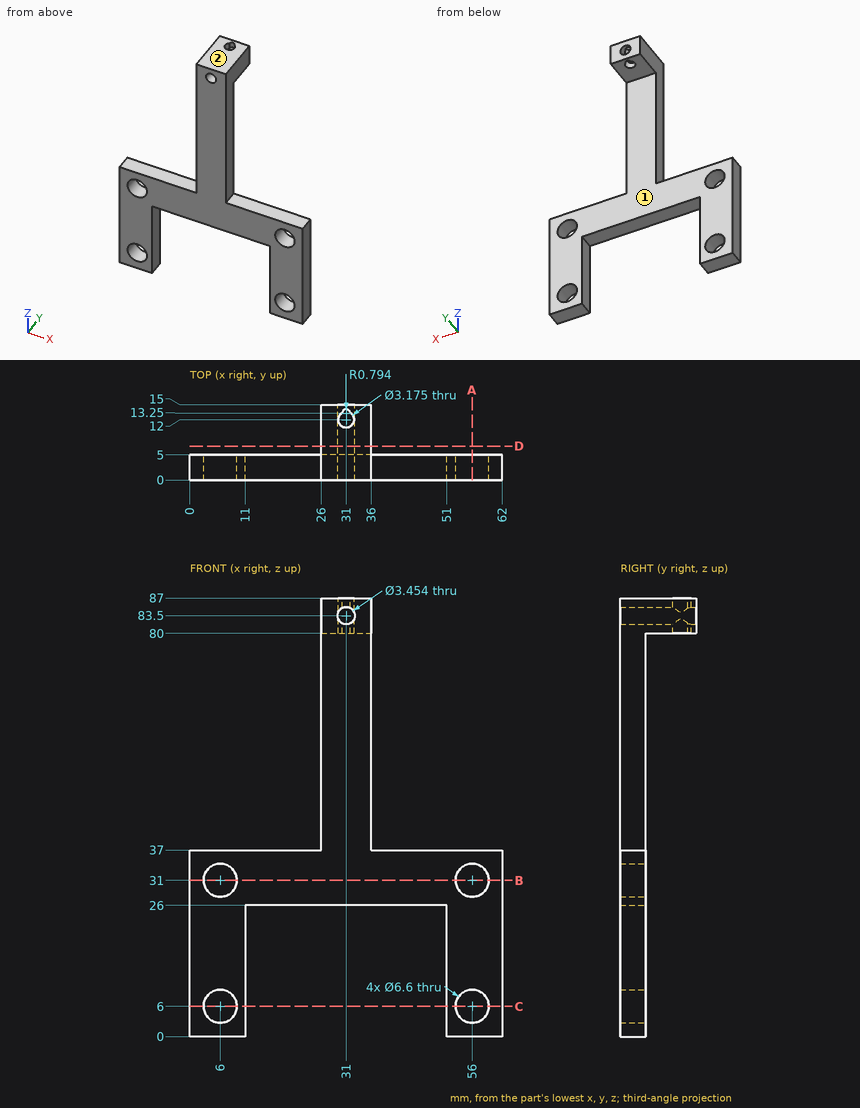
Design review of the part shown in the three views and the two pictorial views. Dimensions are in mm from the part's minimum x, y and z. A direction names the side the tool comes from. Give positions to 0.01 mm unless a question says otherwise; leave off trailing zeros. Loops run counter-clockwise (first coordinate to the right, second up) from the corner with the lowest first, then second, coordinate; pieces in that order, holes last. Notation, with made-up numbers: (-7, 55) - (-3, 55) arc R31 ccw to (-3, 83) - close; hole circle Ø2 at (-19, 81.5). An arc over 180 degrees is marked (long way). Answer as a JSON object with one key per item and string values.
Q1. Add section D-D on y = 6.75. State the section outline as (x, z) points (1 decimal).
Worked out:
{"outline": "(26, 80) - (36, 80) - (36, 87) - (26, 87) - close; hole circle Ø3.5 at (31, 83.5)"}
Q2. For the marked faces 1 and 2, list the 3-axis set-ups (+Z, -Z, +X, -X, +Y, -Y) from which the entire face can be reached by the end or side of a thin tool; tool diameter is ignored.
Worked out:
{"face 1": "-Z, +X, -X, +Y", "face 2": "+Z, +X, -X, +Y, -Y"}
Q3. To check wall thickness, follow line 1 along X through (y, z) = (4.05, 6); line 2 along Z through (x, y) = (6, 2.3); line 3 along X through (y, z) = (2.3, 31). State the ranges of each line that lie inside material, in increasing order.
Worked out:
{"line 1": "x = 0 to 2.7, 9.3 to 11, 51 to 52.7, 59.3 to 62", "line 2": "z = 0 to 2.7, 9.3 to 27.7, 34.3 to 37", "line 3": "x = 0 to 2.7, 9.3 to 52.7, 59.3 to 62"}
Q4. Add section B-B on z = 31. State the section outline as (x, y) points.
Worked out:
{"outline": "(0, 0) - (2.7, 0) - (2.7, 5) - (0, 5) - close; (9.3, 0) - (52.7, 0) - (52.7, 5) - (9.3, 5) - close; (59.3, 0) - (62, 0) - (62, 5) - (59.3, 5) - close"}
Q5. Insertion check: pin 1 (8.5 mm diameter, centred on x = 56, z = 31, fed in from +Y); pin 2 (3 mm diameter, centred on x = 30.5, y = 8.5, fed in from -Z); pin 3 (5.5 mm diameter, centred on x = 46, y = 2, fed in from +Z). Each pin has a flat end and moves straight along its axis. Give the tip position at first contact, or say it passes through.
Worked out:
{"pin 1": "stops at y = 5", "pin 2": "stops at z = 80", "pin 3": "stops at z = 37"}
Q6. Add section C-C on z = 6. State the section outline as (x, y) points, plus the area to 3 significant figures.
Worked out:
{"outline": "(0, 0) - (2.7, 0) - (2.7, 5) - (0, 5) - close; (9.3, 0) - (11, 0) - (11, 5) - (9.3, 5) - close; (51, 0) - (52.7, 0) - (52.7, 5) - (51, 5) - close; (59.3, 0) - (62, 0) - (62, 5) - (59.3, 5) - close", "area": "44.0 mm^2"}
Q7. Add section A-A on x = 56. State the section outline as (y, z) points, plus the area to 3 significant figures.
Worked out:
{"outline": "(0, 0) - (5, 0) - (5, 2.7) - (0, 2.7) - close; (0, 9.3) - (5, 9.3) - (5, 27.7) - (0, 27.7) - close; (0, 34.3) - (5, 34.3) - (5, 37) - (0, 37) - close", "area": "119 mm^2"}
